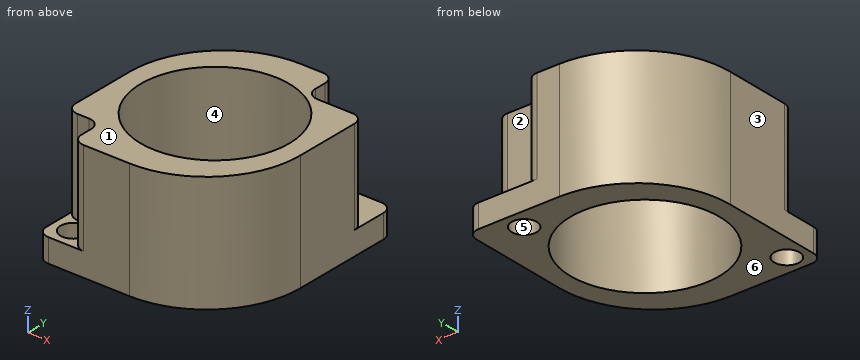
```python
from build123d import *

# Parameters (mm, degrees)
F0_W      = 20.193
F0_H      = 22.352
F1_DEPTH  = 12.7
F2_R      = 8.0645
F3_DEPTH  = 12.7
F5_W      = 3.81
F5_H      = 3.81
F6_DEPTH  = 10.16
F4_W      = 6.35
F4_H      = 3.81
F7_DEPTH  = 10.16
F8_R      = 10.16
F9_R      = 1.27
F11_R     = 1.3716
F12_DEPTH = 2.54
F10_R     = 1.3716
F13_DEPTH = 2.54


with BuildPart() as f1:
    # F0 (on Top) → F1 (new body)
    with BuildSketch(Plane.XY):
        Rectangle(F0_W, F0_H)
    extrude(amount=F1_DEPTH)

    # F2 (on face) → F3 (cut)
    with BuildSketch(Plane.XY.offset(12.7)):
        Circle(F2_R)
    extrude(amount=-F3_DEPTH, mode=Mode.SUBTRACT)

    # F5 (on face) → F6 (cut)
    with BuildSketch(Plane.XY.offset(12.7)):
        with Locations((-8.1915, -9.271)):
            Rectangle(F5_W, F5_H)
    extrude(amount=-F6_DEPTH, mode=Mode.SUBTRACT)

    # F4 (on face) → F7 (cut)
    with BuildSketch(Plane.XY.offset(12.7)):
        with Locations((6.9215, 9.271)):
            Rectangle(F4_W, F4_H)
    extrude(amount=-F7_DEPTH, mode=Mode.SUBTRACT)

    # F8
    f8_edges = [f1.edges().sort_by_distance(p)[0] for p in [
        (-10.0965, 11.176, 6.35),
        (10.0965, -11.176, 6.35),
    ]]
    fillet(f8_edges, radius=F8_R)

    # F9
    f9_edges = [f1.edges().sort_by_distance(p)[0] for p in [
        (-10.0965, -7.366, 7.62),
        (-6.2865, -11.176, 7.62),
        (3.7465, 11.176, 7.62),
        (10.0965, 7.366, 7.62),
        (3.7465, 7.366, 7.62),
        (-6.2865, -7.366, 7.62),
        (-10.0965, -11.176, 1.27),
        (10.0965, 11.176, 1.27),
    ]]
    fillet(f9_edges, radius=F9_R)

    # F11 (on face) → F12 (cut)
    with BuildSketch(Plane.XY.offset(2.54)):
        with Locations((-7.9375, -9.017)):
            Circle(F11_R)
    extrude(amount=-F12_DEPTH, mode=Mode.SUBTRACT)

    # F10 (on face) → F13 (cut)
    with BuildSketch(Plane.XY.offset(2.54)):
        with Locations((5.6515, 9.017)):
            Circle(F10_R)
    extrude(amount=-F13_DEPTH, mode=Mode.SUBTRACT)


solid = f1.part
```
Part model, mm, in its own coordinate system. Face numbers are marked on the shaded views. A direction names the side the tool comes from. Coordinates: 2 decimals unless noted, no trailing zeros. Loops run counter-clockwise (first coordinate to the right, second up) from the corner with the lowest first, then second, coordinate; pieces in that order, holes last. Notation, with made-up numbers: (76, -32) - (135, -32) arc R25 ccw to (135, -7) - close; hole circle Ø6 at (-19.5, -5.75). An arc over 180 degrees is marked (long way). Write item = value, one per line. Start each with the question number.
Item 1: 3-axis set-ups, long thin cutter, end or side, ignore diameter. For the marked faces 1 and 2: which of +Z, -Z, +X, -X, +Y, -Y reach the whole face in a straight line?
Item 2: Wall check: L1, parallel to Y at x = 0, z = 3.5; L2, parallel to X at y = -0.25, z = 7.5; L3, parallel to Y at x = -0.5, z = 9.75. Give the ranges that are in metal, low to high. Write a range as from..to.
Item 3: Mould opens along X. For the marked faces 3, 4, 5 and 6 say: released by +X, released by -X, zero draft, split by the parting line, or undercut.
Item 4: Flat gauge pins, fed straight in: pin 1 Ø3 at (y, z) = (-5.5, 2) entering from +X; pin 2 Ø1 at (y, z) = (9.5, 9.5) entering from +X; pin 3 Ø2.5 at (x, y) = (-7.94, -9.02) entering from +Z; pin 4 Ø0.6 at (x, z) = (-8, 8) entering from -Y. Where does each tip first touch, or does it go through?
Item 5: Cut at C-C, the plane x = -5.5. Give the cut face in (y, z), and give its area (3 significant figures).
Item 6: Cut at A-A, the plane z = 7. Give the cut face in (x, y).
Item 7: Cut at B-B, the plane y = -5.25. Give the cut face in (x, z).
Item 8: Cut at D-D, the plane y = 0. Give the cut face in (x, z), and give its area (3 significant figures).
The answers:
q1.face_1 = +Z, +X, -X, +Y, -Y
q1.face_2 = +Z, +X, +Y
q2.L1 = -11.18..-8.06, 8.06..11.18
q2.L2 = -10.1..-8.06, 8.06..10.1
q2.L3 = -11.18..-8.05, 8.05..11.16
q3.face_3 = released by -X
q3.face_4 = undercut
q3.face_5 = undercut
q3.face_6 = zero draft
q4.pin_1 = 9.65
q4.pin_2 = 3.75
q4.pin_3 = through
q4.pin_4 = -7.37
q5.outline = (-11.18, 0) - (-5.9, 0) - (-5.9, 12.7) - (-11.08, 12.7) - (-11.08, 2.54) - (-11.18, 2.54) - close; (5.9, 0) - (9.52, 0) - (9.52, 12.7) - (5.9, 12.7) - close
q5.area = 112 mm2
q6.outline = (-10.1, -6.1) arc R1.27 ccw to (-8.83, -7.37) - (-7.56, -7.37) arc R1.27 cw to (-6.29, -8.64) - (-6.29, -9.91) arc R1.27 ccw to (-5.02, -11.18) - (-0.06, -11.18) arc R10.16 ccw to (10.1, -1.02) - (10.1, 6.1) arc R1.27 ccw to (8.83, 7.37) - (5.02, 7.37) arc R1.27 cw to (3.75, 8.64) - (3.75, 9.91) arc R1.27 ccw to (2.48, 11.18) - (0.06, 11.18) arc R10.16 ccw to (-10.1, 1.02) - close; hole circle Ø16.13 at (0, 0)
q7.outline = (-10.1, 0) - (-6.12, 0) - (-6.12, 12.7) - (-10.1, 12.7) - close; (6.12, 0) - (9.17, 0) - (9.17, 12.7) - (6.12, 12.7) - close
q8.outline = (-10.1, 0) - (-8.06, 0) - (-8.06, 12.7) - (-10.1, 12.7) - close; (8.06, 0) - (10.1, 0) - (10.1, 12.7) - (8.06, 12.7) - close
q8.area = 51.6 mm2
